```python
from build123d import *

# Parameters (mm, degrees)
BLANKSKE_W         = 44.45
BLANKSKE_H         = 13.97
BLANK_DEPTH        = 12.7
TOOTHCUTSIM_DEPTH  = 49.293409488
TEETHCUTS_COUNT    = 12
TEETHCUTS_PITCH    = 3.989822665
CUT_EXTRUDE1_REACH = 50.293
SKETCH1_R          = 2.4892


with BuildPart() as part:
    # BlankSke → Blank (new body)
    with BuildSketch(Plane.XY):
        with Locations((22.225, 6.985)):
            Rectangle(BLANKSKE_W, BLANKSKE_H)
    extrude(amount=-BLANK_DEPTH)

    # TooCutSkeSim → ToothCutSim (cut, through all)
    with BuildSketch(Plane.XY):
        Polygon((0.595165029, 11.176), (-0.595165029, 11.176), (-1.621342708, 13.9954), (1.621342708, 13.9954), align=None)
    toothcutsim = extrude(amount=-TOOTHCUTSIM_DEPTH, mode=Mode.SUBTRACT)

    # TeethCuts: ToothCutSim ×12
    with Locations(*[(i * TEETHCUTS_PITCH, 0, 0) for i in range(1, TEETHCUTS_COUNT)]):
        add(toothcutsim, mode=Mode.SUBTRACT)

    # Sketch1 → Cut-Extrude1 (cut, up to next)
    with BuildSketch(Plane.XY, mode=Mode.PRIVATE) as cut_extrude1_sk1:
        with Locations((5.08, 5.588)):
            Circle(SKETCH1_R)
    cut_extrude1_tool1 = extrude(cut_extrude1_sk1.sketch, amount=-CUT_EXTRUDE1_REACH, mode=Mode.PRIVATE) & part.part
    add(cut_extrude1_tool1.solids().sort_by_distance((5.08, 5.588, 0))[0], mode=Mode.SUBTRACT)


solid = part.part
```
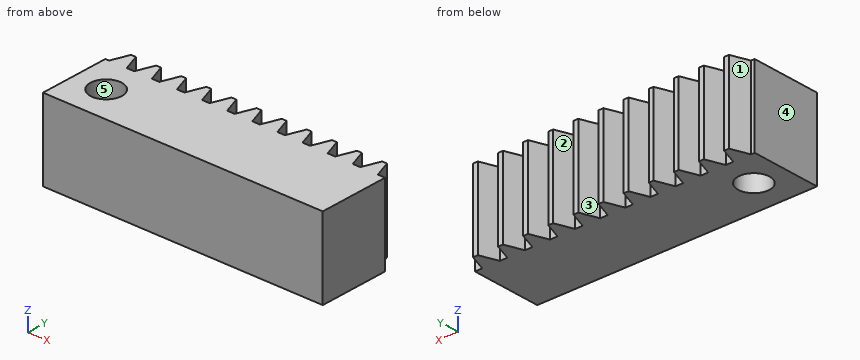
Work out the finished part from the listing and answer in its coordinate system (mm). Face numbers are marked on the shaded views. A direction names the side the tool comes from. Coordinates: 2 decimals unless noted, no trailing zeros. Loops run counter-clockwise (first coordinate to the right, second up) from the corner with the lowest first, then second, coordinate; pieces in that order, holes last.
1) Section B-B (y = 4.5) is taken. Give the vertices of the cut face in (x, z).
Results:
outline: (0, -12.7) - (2.84, -12.7) - (2.84, 0) - (0, 0) - close; (7.32, -12.7) - (44.45, -12.7) - (44.45, 0) - (7.32, 0) - close
2) Section C-C (x = 32) is taken. Give the vertices of the cut face in (y, z), plus the area to 3 significant figures.
Results:
outline: (0, -12.7) - (11.18, -12.7) - (11.18, 0) - (0, 0) - close
area: 142 mm2
3) For a pull along Y with two mould halves and no side action, classify the marked faces 3, 4 and 5 as +Y half, -Y half, draft (parallel to the pull), parting line (faces both ways), or undercut.
Results:
face 3: +Y half
face 4: draft
face 5: undercut
4) Consider probe 1 along X at (y, z) = (4, -3.5); probe 2 along Y at (x, z) = (16, -1.5); probe 3 along X at (y, z) = (3.75, -4). Determine where each line is inside the solid, lowest interval first.
Results:
probe 1: x = 0 to 3.16, 7 to 44.45
probe 2: y = 0 to 11.18
probe 3: x = 0 to 3.4, 6.76 to 44.45
5) For the marked faces 1 and 2, determine the directions among +Z, -Z, +X, -X, +Y, -Y from which every point of the face is accessible in a straight line to the end or side of a thin tool.
Results:
face 1: +Z, -Z, -X, +Y
face 2: +Z, -Z, +Y
6) Flat-ended cylindrical pins translate along their axes: pin 1 (1 mm diameter, centred on x = 12, z = -5, fed in from +Y); pin 2 (4 mm diameter, centred on x = 5.08, y = 5.588, fed in from +Z). Find the tip coordinate at first contact, or state that the pin passes through.
Results:
pin 1: stops at y = 11.18
pin 2: passes through
7) Section A-A (x = 5.08) is taken. Give the vertices of the cut face in (y, z), plus the area to 3 significant figures.
Results:
outline: (0, -12.7) - (3.1, -12.7) - (3.1, 0) - (0, 0) - close; (8.08, -12.7) - (12.54, -12.7) - (12.54, 0) - (8.08, 0) - close
area: 96.0 mm2
